from build123d import *

# Parameters (mm, degrees)
MODEL_R                 = 8
MODEL_W                 = 10
MODEL_H                 = 2.9
SALIENTE_EXTRUIR1_DEPTH = 3


with BuildPart() as part:
    # Model → Saliente-Extruir1 (new body)
    with BuildSketch(Plane.XY):
        with BuildLine():
            Line((2.738139573, 79.958721833), (1.893307256, 64.837008948))
            ThreePointArc((1.893307256, 64.837008948), (1.804094173, 52.374094451), (8.490003457, 41.855976094))
            ThreePointArc((8.490003457, 41.855976094), (9.866643854, 37.389168926), (6.950289352, 33.736446451))
            ThreePointArc((6.950289352, 33.736446451), (3.525794094, 31.275549631), (1.420223138, 27.621818403))
            ThreePointArc((1.420223138, 27.621818403), (-0.672991735, 13.448943974), (1.903257207, -0.64413445))
            ThreePointArc((1.903257207, -0.64413445), (1.596863178, -1.105922047), (1.627780863, -1.659247614))
            ThreePointArc((1.627780863, -1.659247614), (2.122286511, -1.493378675), (2.468024937, -1.102849184))
            ThreePointArc((2.468024937, -1.102849184), (2.58077221, -1.616114359), (2.813255055, -2.087394334))
            ThreePointArc((2.813255055, -2.087394334), (3.27699089, -1.806143429), (3.602865379, -1.372601258))
            ThreePointArc((3.602865379, -1.372601258), (3.657014656, -1.871943312), (3.909736594, -2.306001204))
            ThreePointArc((3.909736594, -2.306001204), (4.43140284, -2.078027301), (4.811170789, -1.653899872))
            ThreePointArc((4.811170789, -1.653899872), (4.785196909, -2.222836522), (5.02214475, -2.740735426))
            ThreePointArc((5.02214475, -2.740735426), (5.596433055, -2.488050459), (6.0194762, -2.02470259))
            ThreePointArc((6.0194762, -2.02470259), (6.087237768, -2.398385139), (6.345526866, -2.676803923))
            ThreePointArc((6.345526866, -2.676803923), (6.76512344, -2.4701067), (7.016807649, -2.075847793))
            ThreePointArc((7.016807649, -2.075847793), (10.072385436, 5.017714023), (10.480834721, 12.730582753))
            ThreePointArc((10.480834721, 12.730582753), (11.467458305, 9.658521652), (12.192311398, 6.514388466))
            ThreePointArc((12.192311398, 6.514388466), (12.245025503, 5.0311028), (11.859988831, 3.59769361))
            ThreePointArc((11.859988831, 3.59769361), (8.838306655, -6.448503975), (8.27496016, -16.924156212))
            ThreePointArc((8.27496016, -16.924156212), (8.190311904, -18.223316893), (7.773132872, -19.456583068))
            ThreePointArc((7.773132872, -19.456583068), (6.18189197, -22.450615029), (4.403832579, -25.337616899))
            ThreePointArc((4.403832579, -25.337616899), (4.303591918, -25.529024451), (4.164576282, -25.69443211))
            ThreePointArc((4.164576282, -25.69443211), (0.867440919, -30.254572833), (-0.599469924, -35.687266233))
            ThreePointArc((-0.599469924, -35.687266233), (-0.601989014, -35.811902896), (-0.588981272, -35.935884517))
            ThreePointArc((-0.588981272, -35.935884517), (0.978789677, -38.80548638), (3.98481018, -40.092483401))
            ThreePointArc((3.98481018, -40.092483401), (0.856364533, -41.485661692), (-0.680047474, -44.546308039))
            ThreePointArc((-0.680047474, -44.546308039), (0.784377961, -48.081916287), (4.319952525, -49.54642304))
            Line((4.319952525, -49.54642304), (19.820067057, -49.54642304))
            Line((19.820067057, -49.54642304), (19.820067057, -45.54642304))
            Line((19.820067057, -45.54642304), (22.820067057, -45.54642304))
            Line((22.820067057, -45.54642304), (22.820067057, -49.54642304))
            ThreePointArc((22.820067057, -49.54642304), (26.431019228, -47.64752109), (28.47138138, -44.114572394))
            Line((28.47138138, -44.114572394), (35.168752734, -44.114572394))
            ThreePointArc((35.168752734, -44.114572394), (37.209114886, -47.64752109), (40.820067057, -49.54642304))
            Line((40.820067057, -49.54642304), (40.820067057, -45.54642304))
            Line((40.820067057, -45.54642304), (43.820067057, -45.54642304))
            Line((43.820067057, -45.54642304), (43.820067057, -49.54642304))
            Line((43.820067057, -49.54642304), (59.320181589, -49.54642304))
            ThreePointArc((59.320181589, -49.54642304), (62.461382403, -48.436520397), (64.208012382, -45.599566018))
            ThreePointArc((64.208012382, -45.599566018), (63.165796759, -41.825774349), (59.655323933, -40.092483401))
            ThreePointArc((59.655323933, -40.092483401), (62.661344437, -38.80548638), (64.229115385, -35.935884517))
            ThreePointArc((64.229115385, -35.935884517), (64.242123128, -35.811902896), (64.239604038, -35.687266233))
            ThreePointArc((64.239604038, -35.687266233), (62.731421175, -30.274249113), (59.475557832, -25.69443211))
            ThreePointArc((59.475557832, -25.69443211), (59.336542196, -25.529024451), (59.236301535, -25.337616899))
            ThreePointArc((59.236301535, -25.337616899), (57.458242143, -22.450615029), (55.867001242, -19.456583068))
            ThreePointArc((55.867001242, -19.456583068), (55.449822209, -18.223316893), (55.365173954, -16.924156212))
            ThreePointArc((55.365173954, -16.924156212), (54.801827459, -6.448503975), (51.780145282, 3.59769361))
            ThreePointArc((51.780145282, 3.59769361), (51.395108611, 5.0311028), (51.447822716, 6.514388466))
            ThreePointArc((51.447822716, 6.514388466), (52.172675809, 9.658521652), (53.159299392, 12.730582753))
            ThreePointArc((53.159299392, 12.730582753), (53.567748677, 5.017714023), (56.623326464, -2.075847793))
            ThreePointArc((56.623326464, -2.075847793), (56.875010673, -2.4701067), (57.294607248, -2.676803923))
            ThreePointArc((57.294607248, -2.676803923), (57.552896345, -2.398385139), (57.620657914, -2.02470259))
            ThreePointArc((57.620657914, -2.02470259), (58.043701059, -2.488050459), (58.617989364, -2.740735426))
            ThreePointArc((58.617989364, -2.740735426), (58.854937205, -2.222836522), (58.828963324, -1.653899872))
            ThreePointArc((58.828963324, -1.653899872), (59.208731274, -2.078027301), (59.73039752, -2.306001204))
            ThreePointArc((59.73039752, -2.306001204), (59.983119457, -1.871943312), (60.037268735, -1.372601258))
            ThreePointArc((60.037268735, -1.372601258), (60.363143224, -1.806143429), (60.826879059, -2.087394334))
            ThreePointArc((60.826879059, -2.087394334), (61.059361903, -1.616114359), (61.172109176, -1.102849184))
            ThreePointArc((61.172109176, -1.102849184), (61.517847602, -1.493378675), (62.012353251, -1.659247614))
            ThreePointArc((62.012353251, -1.659247614), (62.043270935, -1.105922047), (61.736876906, -0.64413445))
            ThreePointArc((61.736876906, -0.64413445), (63.602383612, 6.292702198), (64.312985392, 13.440769284))
            ThreePointArc((64.312985392, 13.440769284), (63.807919995, 20.611213234), (62.219910975, 27.621818403))
            ThreePointArc((62.219910975, 27.621818403), (60.11434002, 31.275549631), (56.689844761, 33.736446451))
            ThreePointArc((56.689844761, 33.736446451), (53.773490259, 37.389168926), (55.150130657, 41.855976094))
            ThreePointArc((55.150130657, 41.855976094), (61.836039941, 52.374094451), (61.746826857, 64.837008948))
            Line((61.746826857, 64.837008948), (60.901994541, 79.958721833))
            ThreePointArc((60.901994541, 79.958721833), (60.52523779, 81.01221194), (60.082132629, 82.039560406))
            ThreePointArc((60.082132629, 82.039560406), (57.301545651, 86.145115147), (53.573638816, 89.414664704))
            ThreePointArc((53.573638816, 89.414664704), (56.089558762, 91.529262633), (58.501636282, 93.761584207))
            ThreePointArc((58.501636282, 93.761584207), (64.487990723, 100.682191439), (69.3188096, 108.45357696))
            ThreePointArc((69.3188096, 108.45357696), (54.700807458, 103.978782371), (43.444082198, 93.634899654))
            ThreePointArc((43.444082198, 93.634899654), (28.686150355, 95.095319384), (14.288476391, 91.540553218))
            ThreePointArc((14.288476391, 91.540553218), (8.469304852, 101.471337422), (-0.6811904, 108.45357696))
            ThreePointArc((-0.6811904, 108.45357696), (0.464967816, 95.691689927), (4.311825224, 83.469532696))
            ThreePointArc((4.311825224, 83.469532696), (3.428504493, 81.757372515), (2.738139573, 79.958721833))
        make_face()
        with Locations((18.820067057, 68.975620222)):
            Circle(MODEL_R, mode=Mode.SUBTRACT)
        with Locations((44.820067057, 68.975620222)):
            Circle(MODEL_R, mode=Mode.SUBTRACT)
        with Locations((44.320067057, -23.09642304)):
            Rectangle(MODEL_W, MODEL_H, mode=Mode.SUBTRACT)
        with Locations((19.320067057, -23.09642304)):
            Rectangle(MODEL_W, MODEL_H, mode=Mode.SUBTRACT)
        Polygon((32.320067057, 15.131610977), (47.820067057, 15.131610977), (47.820067057, -16.868389023), (15.820067057, -16.868389023), (15.820067057, 15.131610977), align=None, mode=Mode.SUBTRACT)
    extrude(amount=SALIENTE_EXTRUIR1_DEPTH)


solid = part.part
Can you work these out from the model? Positions are in its coordinate system, mm. A direction names the side the tool comes from. Give positions to 0.01 mm unless a question says otherwise; leave off trailing zeros. Order: outer loops, then holes, each group sorted by start corner. A loop starts at its lowest first (then second) coordinate and runs counter-clockwise, first axis right, second up. Notation, with made-up numbers: (-36.5, -32) - (-28.5, -32) arc R17 cw to (-28.5, -2) - close; hole circle Ø7 at (23, 55.25). An arc over 180 degrees is marked (long way). Write each question's results on one line, items separated by ' | '.
1) Please list where these lines run through material, in increasing order: line 1 along Y through (x, z) = (57, 0.7); line 2 along Y through (x, z) = (14.5, 2.9); line 3 along Y through (x, z) = (56, 0.45). Write a range as [from, to].
Final values:
line 1: y = [-49.55, -21.63], [-2.56, 33.6], [43.67, 86.48], [92.35, 105.18] | line 2: y = [-49.55, -24.55], [-21.65, 62.24], [75.71, 91.63] | line 3: y = [-49.55, -19.73], [-1.07, 34.1], [42.64, 87.48], [91.45, 104.69]
2) If we mould it in two halves opening along X, with no side actions, what happens to faces 5 (the face through (6.205, -22.409, 1.479)), 6 (the face through (61.787, 52.204, 1.479)), 7 (the face through (8.576, 101.35, 1.479))? For each: pulls with the +X half, pulls with the -X half, needs draft (parallel to the pull), parting line crosses it, or undercut.
Final values:
face 5: pulls with the -X half | face 6: pulls with the +X half | face 7: undercut
3) I'm going to push flat-ended pins straight in: pin 1 Ø1.5 at (x, z) = (22, 1) entering from -Y; pin 2 Ø12 at (x, y) = (20.5, 3.5) entering from +Z; pin 3 Ø0.9 at (y, z) = (-47.5, 1.5) entering from +X; pin 4 Ø0.9 at (y, z) = (-2, 2) entering from +X. Where does each tip first touch, or does it pass through?
Final values:
pin 1: stops at y = -45.55 | pin 2: stops at z = 3 | pin 3: stops at x = 63.65 | pin 4: stops at x = 62.05
4) Suppose I cut it at D-D, the plane y = 44. Write out the boundary of the cut face in (x, z), then the cut area to 3 significant figures.
Final values:
outline: (6.35, 0) - (57.29, 0) - (57.29, 3) - (6.35, 3) - close | area: 153 mm^2
5) On a 3-axis mill with a long thin cutter (end or side, diameter ignored), from which of +Z, -Z, +X, -X, +Y, -Y can I reach the whole of each face in a straight line? I mean faces 1 (the face through (40.82, -48, 1)), 2 (the face through (60.154, 31.231, 1.479)), 3 (the face through (54.888, 104.085, 1.479)), 4 (the face through (14.32, -23, 1)). Say none if no direction works.
Final values:
face 1: +Z, -Z, -Y | face 2: +Z, -Z, +X | face 3: +Z, -Z, +Y | face 4: +Z, -Z
6) Suppose I cut it at A-A, the plane y = 67.5. Write out the boundary of the cut face in (x, z).
Final values:
outline: (2.04, 0) - (10.96, 0) - (10.96, 3) - (2.04, 3) - close; (26.68, 0) - (36.96, 0) - (36.96, 3) - (26.68, 3) - close; (52.68, 0) - (61.6, 0) - (61.6, 3) - (52.68, 3) - close
7) Suppose I cut it at B-B, the plane y = 17. Write out the boundary of the cut face in (x, z), then the cut area to 3 significant figures.
Final values:
outline: (-0.59, 0) - (64.2, 0) - (64.2, 3) - (-0.59, 3) - close | area: 194 mm^2
8) Suppose I cut it at C-C, the plane z = 1.7. Give the number of separate pieces and of enclosed holes in the cut face, then the cut area to 3 significant figures.
Final values:
separate pieces: 1 | enclosed holes: 5 | area: 6,900 mm^2
